```python
from build123d import *

# Parameters (mm, degrees)
SKETCH1_R               = 8.3
BOSS_EXTRUDE1_DEPTH     = 1.8
BOSS_EXTRUDE2_DEPTH     = 82.75
SKETCH3_R               = 7.25
BOSS_EXTRUDE3_DEPTH     = 1.15
SKETCH4_R               = 7.55
BOSS_EXTRUDE4_DEPTH     = 6.7
CHAMFER1_SIZE           = 2.023
CHAMFER1_SIZE2          = 7.549938784
CUT_EXTRUDE1_DEPTH      = 2
CUT_EXTRUDE1_DEPTH_BACK = 2
CUT_EXTRUDE2_DEPTH      = 2
CUT_EXTRUDE2_DEPTH_BACK = 2


with BuildPart() as part:
    # Sketch1 → Boss-Extrude1 (new body)
    with BuildSketch(Plane(origin=(0, 0, 0), x_dir=(1, 0, 0), z_dir=(0, 1, 0))):
        with Locations(Location((0, 0, 0), (0, 0, 270))):
            Circle(SKETCH1_R)
    extrude(amount=BOSS_EXTRUDE1_DEPTH)

    # Sketch2 → Boss-Extrude2 (add)
    with BuildSketch(Plane(origin=(0, 1.8, 0), x_dir=(1, 0, 0), z_dir=(0, 1, 0))):
        Polygon((-0.475, 0.475), (-0.475, 7), (0.475, 7), (0.475, 0.475), (7, 0.475), (7, -0.475), (0.475, -0.475), (0.475, -7), (-0.475, -7), (-0.475, -0.475), (-7, -0.475), (-7, 0.475), align=None)
    extrude(amount=BOSS_EXTRUDE2_DEPTH)

    # Sketch3 → Boss-Extrude3 (add)
    with BuildSketch(Plane(origin=(0, 84.55, 0), x_dir=(1, 0, 0), z_dir=(0, 1, 0))):
        with Locations(Location((0, 0, 0), (0, 0, 270))):
            Circle(SKETCH3_R)
    extrude(amount=BOSS_EXTRUDE3_DEPTH)

    # Sketch4 → Boss-Extrude4 (add)
    with BuildSketch(Plane(origin=(0, 85.7, 0), x_dir=(1, 0, 0), z_dir=(0, 1, 0))):
        with Locations(Location((0, 0, 0), (0, 0, 270))):
            Circle(SKETCH4_R)
    extrude(amount=BOSS_EXTRUDE4_DEPTH)

    # Chamfer1
    chamfer1_edges = [part.edges().sort_by_distance(p)[0] for p in [
        (0, 92.4, -7.55),
    ]]
    chamfer1_side = [part.faces().sort_by_distance(p)[0] for p in [
        (0, 89.05, -7.55),
    ]]
    chamfer(chamfer1_edges, length=CHAMFER1_SIZE, length2=CHAMFER1_SIZE2, reference=chamfer1_side[0])

    # Sketch7 → Cut-Extrude1 (cut, two sides: drawn at the far end of the back side and taken through both)
    with BuildSketch(Plane(origin=(0.475, 0, 0), x_dir=(0, 0, -1), z_dir=(1, 0, 0)).offset(-CUT_EXTRUDE1_DEPTH_BACK)):
        with BuildLine():
            Line((-7, 1.8), (-7, 23.65))
            add(Edge.make_bspline(
                [(-5.125, 18.3), (-5.059549187, 21.3387368), (-7, 23.65)],
                knots=[0, 0, 0, 1, 1, 1], degree=2))
            Line((-5.125, 18.3), (-5.125, 1.8))
            Line((-5.125, 1.8), (-7, 1.8))
        make_face()
        with BuildLine():
            Line((5.125, 1.8), (5.125, 18.3))
            add(Edge.make_bspline(
                [(5.125, 18.3), (5.059549187, 21.3387368), (7, 23.65)],
                knots=[0, 0, 0, 1, 1, 1], degree=2))
            Line((7, 23.65), (7, 1.8))
            Line((7, 1.8), (5.125, 1.8))
        make_face()
    extrude(amount=CUT_EXTRUDE1_DEPTH + CUT_EXTRUDE1_DEPTH_BACK, mode=Mode.SUBTRACT)

    # Sketch8 → Cut-Extrude2 (cut, two sides: drawn at the far end of the back side and taken through both)
    with BuildSketch(Plane.XY.offset(-CUT_EXTRUDE2_DEPTH_BACK)):
        with BuildLine():
            Line((-7, 1.8), (-7, 23.65))
            add(Edge.make_bspline(
                [(-5.125, 18.3), (-5.02840034, 21.345891772), (-7, 23.65)],
                knots=[0, 0, 0, 1, 1, 1], degree=2))
            Line((-5.125, 18.3), (-5.125, 1.8))
            Line((-5.125, 1.8), (-7, 1.8))
        make_face()
        with BuildLine():
            Line((7, 1.8), (5.125, 1.8))
            Line((5.125, 1.8), (5.125, 18.3))
            add(Edge.make_bspline(
                [(5.125, 18.3), (5.02840034, 21.345891772), (7, 23.65)],
                knots=[0, 0, 0, 1, 1, 1], degree=2))
            Line((7, 23.65), (7, 1.8))
        make_face()
    extrude(amount=CUT_EXTRUDE2_DEPTH + CUT_EXTRUDE2_DEPTH_BACK, mode=Mode.SUBTRACT)


solid = part.part
```
The listing builds one solid part. Answer for the finished solid, in the listing's coordinates (mm). A direction names the side the tool comes from. Coordinates: 2 decimals unless noted, no trailing zeros. Loops run counter-clockwise (first coordinate to the right, second up) from the corner with the lowest first, then second, coordinate; pieces in that order, holes last. Notation, with made-up numbers: (50, 28) -> (55, 28) arc R28 ccw to (55, 54) -> close; hole circle Ø10 at (46.25, -33.75). An arc over 180 degrees is marked (long way). Use one line per item in the form item = value. Start each with the question number.
Item 1: Consider L1, parallel to Z at x = 1, y = 6.5 (3 decimals); L2, parallel to X at y = 70, z = 0. Determine where each line is inside the solid, lowest interval first. Write a range as [from, to].
Item 2: The part is cut by section A-A on y = 57.5. Determine the outline of the cut face in (x, z) (3 decimals), then the cut area to 3 significant figures.
Item 3: A tool of negligible diameter and unlimited length cuts with its end or side. For faces 1 (the face through (0.475, 43, -4)), 2 (the face through (-4, 43, 0.475)), 3 (the face through (-2.777, 85.117, 6.697)), from which of +Z, -Z, +X, -X, +Y, -Y can it reach the whole face along a straight path? Write none if from no direction.
Item 4: Flat-ended cylindrical pins translate along their axes: pin 1 Ø0.8 at (x, y) = (0, 56) entering from +Z; pin 2 Ø2 at (y, z) = (52, -4.5) entering from -X (3 decimals); pin 3 Ø5 at (x, y) = (-4.5, 34) entering from -Z (3 decimals). Find the tip coordinate at first contact, or state that the pin passes through.
Item 5: The mould has two halves that part along Y. Classify faces 4 (the face through (0, 0, 0)), 5 (the face through (0.475, 43, 4)), 6 (the face through (4, 43, 0.475)), 7 (the face through (-5.05, 0.887, -6.587)): released by +Y, released by -Y, zero draft, split by the parting line, or undercut.
Answer key:
q1.L1 = [-0.475, 0.475]
q1.L2 = [-7, 7]
q2.outline = (-7, -0.475) -> (-0.475, -0.475) -> (-0.475, -7) -> (0.475, -7) -> (0.475, -0.475) -> (7, -0.475) -> (7, 0.475) -> (0.475, 0.475) -> (0.475, 7) -> (-0.475, 7) -> (-0.475, 0.475) -> (-7, 0.475) -> close
q2.area = 25.7 mm2
q3.face_1 = -Z, +X
q3.face_2 = +Z, -X
q3.face_3 = none
q4.pin_1 = 7
q4.pin_2 = -0.475
q4.pin_3 = -0.475
q5.face_4 = released by -Y
q5.face_5 = undercut
q5.face_6 = undercut
q5.face_7 = zero draft
